Check sheet for the modelled part. Datum: model origin and axes. Units: mm. Face numbers are marked on the shaded views. Round coordinates to 2 decimals unless told otherwise and drop trailing zeros. Loops run counter-clockwise (first coordinate to the right, second up) from the corner with the lowest first, then second, coordinate; pieces in that order, holes last. Notation, with made-up numbers: (69.25, 30.5) - (114.25, 30.5) arc R31 ccw to (114.25, 55.5) - close; hole circle Ø5 at (-18, 65). An arc over 180 degrees is marked (long way). Answer in a Markdown table with one row per item. Add a question column.
(1) Mould release check, pull along X, two halves, no side actions. Record for the marked faces 1, 2, 3 and 4: +X half, -X half, draft (parallel to the pull), parting line (faces both ways), or undercut.
(2) Cross-section at D-D on z = -15. Enter the section's corners in (x, y).
(3) Cross-section at B-B on y = 6.5. Count the separate pieces of the cut face and the enclosed holes in it, then the cut area to 3 significant figures.
(4) Thickness scan on line 1 along Z through (x, y) = (23, 2.75); line 2 along Z through (x, y) = (5, 3.25); line 3 along X through (y, z) = (9.75, -5). Record the ranges inside material, lowest first.
(5) Gauge pin test, flat ends, axial feed: pin 1 (8 mm diameter, centred on x = 13, z = -6.5, fed in from +Y); pin 2 (1 mm diameter, centred on x = 43.5, y = 5.5, fed in from +Z). Record the tip position at first contact, or that the pin passes through.
(6) Cross-section at A-A on x = 45. Enter the section's corners in (y, z).
(7) Cross-section at C-C on x = 33. Enter the section's corners in (y, z).
from build123d import *

# Parameters (mm, degrees)
SKETCH1_W           = 50
SKETCH1_H           = 36
SKETCH1_R           = 4.5
SKETCH1_R_2         = 1.7
BOSS_EXTRUDE1_DEPTH = 12.7


with BuildPart() as part:
    # Sketch1 → Boss-Extrude1 (new body)
    with BuildSketch(Plane(origin=(0, 0, 0), x_dir=(1, 0, 0), z_dir=(0, 1, 0))):
        with Locations((25, 18)):
            Rectangle(SKETCH1_W, SKETCH1_H)
        with Locations((13, 6.5)):
            Circle(SKETCH1_R, mode=Mode.SUBTRACT)
        with Locations((5, 5)):
            Circle(SKETCH1_R_2, mode=Mode.SUBTRACT)
        with Locations((5, 31)):
            Circle(SKETCH1_R_2, mode=Mode.SUBTRACT)
        with Locations((45, 31)):
            Circle(SKETCH1_R_2, mode=Mode.SUBTRACT)
        with Locations((45, 5)):
            Circle(SKETCH1_R_2, mode=Mode.SUBTRACT)
        with Locations((23, 6.5)):
            Circle(SKETCH1_R, mode=Mode.SUBTRACT)
        with Locations((33, 6.5)):
            Circle(SKETCH1_R, mode=Mode.SUBTRACT)
        with Locations((23, 16.5)):
            Circle(SKETCH1_R, mode=Mode.SUBTRACT)
        with Locations((33, 16.5)):
            Circle(SKETCH1_R, mode=Mode.SUBTRACT)
        with Locations((23, 26.5)):
            Circle(SKETCH1_R, mode=Mode.SUBTRACT)
        with Locations((33, 26.5)):
            Circle(SKETCH1_R, mode=Mode.SUBTRACT)
        with Locations((13, 16.5)):
            Circle(SKETCH1_R, mode=Mode.SUBTRACT)
        with Locations((13, 26.5)):
            Circle(SKETCH1_R, mode=Mode.SUBTRACT)
    extrude(amount=BOSS_EXTRUDE1_DEPTH)


solid = part.part
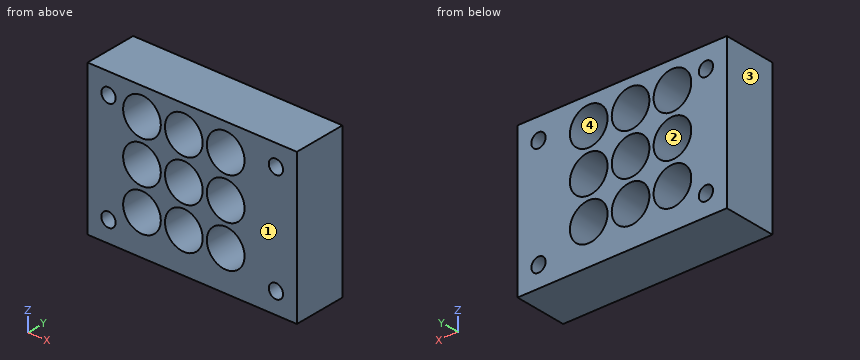
Answers:
| question | item | result |
|---|---|---|
| 1 | face 1 | draft |
| 1 | face 2 | undercut |
| 1 | face 3 | -X half |
| 1 | face 4 | undercut |
| 2 | outline | (0, 0) - (8.76, 0) - (8.76, 12.7) - (0, 12.7) - close; (17.24, 0) - (18.76, 0) - (18.76, 12.7) - (17.24, 12.7) - close; (27.24, 0) - (28.76, 0) - (28.76, 12.7) - (27.24, 12.7) - close; (37.24, 0) - (50, 0) - (50, 12.7) - (37.24, 12.7) - close |
| 3 | separate pieces | 1 |
| 3 | enclosed holes | 13 |
| 3 | area | 1,190 mm^2 |
| 4 | line 1 | z = -36 to -31, -22 to -21, -12 to -11, -2 to 0 |
| 4 | line 2 | z = -36 to -32.7, -29.3 to -6.7, -3.3 to 0 |
| 4 | line 3 | x = 0 to 3.3, 6.7 to 8.76, 17.24 to 18.76, 27.24 to 28.76, 37.24 to 43.3, 46.7 to 50 |
| 5 | pin 1 | passes through |
| 5 | pin 2 | stops at z = 0 |
| 6 | outline | (0, -36) - (12.7, -36) - (12.7, -32.7) - (0, -32.7) - close; (0, -29.3) - (12.7, -29.3) - (12.7, -6.7) - (0, -6.7) - close; (0, -3.3) - (12.7, -3.3) - (12.7, 0) - (0, 0) - close |
| 7 | outline | (0, -36) - (12.7, -36) - (12.7, -31) - (0, -31) - close; (0, -22) - (12.7, -22) - (12.7, -21) - (0, -21) - close; (0, -12) - (12.7, -12) - (12.7, -11) - (0, -11) - close; (0, -2) - (12.7, -2) - (12.7, 0) - (0, 0) - close |
